For this review, take the finished solid that the model builds, in its own axes (mm). A direction names the side the tool comes from. Coordinates: 2 decimals unless noted, no trailing zeros. Write each loop counter-clockwise with the first axis right and the second up, starting at its lowest first coordinate (ties: lowest second). Pieces come first, ordered by that corner, then holes. Notation, with made-up numbers: (78.5, 47.25) -> (87.5, 47.25) arc R32 ccw to (87.5, 77.25) -> close; hole circle Ø1 at (-19.5, 25.5). An arc over 180 degrees is marked (long way). One line per item, written item: value. Start each with the question number.
1) Machinability: for faces 4 (the flat face through (6.9, 46.25, 26.11)), 5 (the cylindrical face through (4.14, 5.1, 6.08)), 6 (the flat face through (36, 25, 23)), which of the approach directions +Z, -Z, +X, -X, +Y, -Y give a long, thin tool a straight path to every point of the face, cutting with its end or side? Answer none if there is none.
2) For pin 1 Ø9.5 at (x, y) = (7, 6) entering from +Z; pin 2 Ø3 at (x, z) = (9.5, 9.5) entering from -Y; pin 3 Ø5 at (x, y) = (7, 44) entering from -Z; pin 4 Ø1 at (x, y) = (27.5, 24) entering from +Z, all flat-tipped, find the tip position at first contact; note any pin that passes through.
3) For probe 1 along Y at (x, z) = (7, 8); probe 2 along X at (y, z) = (44, 9.25); probe 3 along Z at (x, y) = (10, 25), list the stretches that pass through material, from the lowest coordinate up. Write a range as from..to.
4) Add section A-A (y = 25). State the section outline as (x, z) points.
5) Add section C-C (z = 36). State the section outline as (x, y) points.
6) Mouldability with a two-part tool opening along X and no side actions: class faces 1 (the conical face through (7.3, 5.6, 13.5)), 2 (the flat face through (6.902, 3.855, 26.511)), 3 (the flat face through (50, 25, 21)) as released by +X, released by -X, zero draft, split by the parting line, or undercut.
7) Add section D-D (z = 17.5). State the section outline as (x, y) points.
8) Add section B-B (x = 38.5). State the section outline as (y, z) points, and give its area (3 significant figures).
from build123d import *

# Parameters (mm, degrees)
F0_R     = 10
F1_DEPTH = 50
F2_W     = 22
F2_H     = 51.6468636014
F3_DEPTH = 61.9
F5_D     = 6
F5_DEPTH = 12
F5_TIP   = 1.8025818571


with BuildPart() as f1:
    # F0 (on Right) → F1 (new body)
    with BuildSketch(Plane.YZ):
        with BuildLine():
            Line((0, 12), (0, 0))
            Line((0, 0), (50, 0))
            Line((50, 0), (50, 12))
            Line((50, 12), (42.3966097096, 40.6214684475))
            ThreePointArc((42.3966097096, 40.6214684475), (25, 54), (7.6033902904, 40.6214684475))
            Line((7.6033902904, 40.6214684475), (0, 12))
        make_face()
        with Locations((25, 36)):
            Circle(F0_R, mode=Mode.SUBTRACT)
    extrude(amount=F1_DEPTH)

    # F2 (on face) → F3 (cut)
    with BuildSketch(Plane(origin=(0, 50, 0), x_dir=(-1, 0, 0), z_dir=(0, 1, 0))):
        with Locations((-25, 37.8234318007)):
            Rectangle(F2_W, F2_H)
    extrude(amount=-F3_DEPTH, mode=Mode.SUBTRACT)

    # F5
    with Locations(Plane(origin=(0, 0, 0), x_dir=(1, 0, 0), z_dir=(0, 0, -1))):
        with Locations((7, -6), (7, -44), (43, -44), (43, -6)):
            Hole(F5_D / 2, depth=F5_DEPTH)
            with Locations((0, 0, -(F5_DEPTH + F5_TIP / 2))):  # 118° drill point
                Cone(0, F5_D / 2, F5_TIP, mode=Mode.SUBTRACT)


solid = f1.part
Numbers:
1. face 4: +Z, +X, -X, +Y
1. face 5: -Z
1. face 6: +Z, +Y, -Y
2. pin 1: z = 47
2. pin 2: y = 0
2. pin 3: z = 12.3
2. pin 4: z = 12
3. probe 1: 0..3, 9..41, 47..50
3. probe 2: 0..4, 10..40, 46..50
3. probe 3: 0..26, 46..54
4. outline: (0, 0) -> (50, 0) -> (50, 26) -> (36, 26) -> (36, 12) -> (14, 12) -> (14, 26) -> (0, 26) -> close; (0, 46) -> (14, 46) -> (14, 54) -> (0, 54) -> close; (36, 46) -> (50, 46) -> (50, 54) -> (36, 54) -> close
5. outline: (0, 6.38) -> (14, 6.38) -> (14, 15) -> (0, 15) -> close; (0, 35) -> (14, 35) -> (14, 43.62) -> (0, 43.62) -> close; (36, 6.38) -> (50, 6.38) -> (50, 15) -> (36, 15) -> close; (36, 35) -> (50, 35) -> (50, 43.62) -> (36, 43.62) -> close
6. face 1: undercut
6. face 2: zero draft
6. face 3: released by +X
7. outline: (0, 1.46) -> (14, 1.46) -> (14, 48.54) -> (0, 48.54) -> close; (36, 1.46) -> (50, 1.46) -> (50, 48.54) -> (36, 48.54) -> close
8. outline: (0, 0) -> (50, 0) -> (50, 12) -> (42.4, 40.62) arc R18 ccw to (7.6, 40.62) -> (0, 12) -> close; hole circle Ø20 at (25, 36)
8. area: 1,840 mm²
